from build123d import *

# Parameters (mm, degrees)
SKETCH_1_R          = 20
SKETCH_1_R_2        = 15
EXTRUDE_1_DEPTH     = 4
SKETCH_1_3_R        = 15
EXTRUDE_2_DEPTH     = 15
EXTRUDE_START       = 4
SKETCH_2_R          = 20
EXTRUDE_3_DEPTH     = 4
SKETCH_3_R          = 10
SKETCH_3_R_2        = 4
EXTRUDE_4_DEPTH     = 12
CUT_EXTRUDE_1_DEPTH = 18
CUT_EXTRUDE_START   = -27
SKETCH_3_3_R        = 4
CUT_EXTRUDE_2_DEPTH = 27


with BuildPart() as part:
    # Sketch 1 → Extrude 1 (new body)
    # profile 1 of 2: a face of its own
    with BuildSketch(Plane.XY):
        Circle(SKETCH_1_R)
        Circle(SKETCH_1_R_2, mode=Mode.SUBTRACT)
    # profile 2 of 2: a face of its own
    with BuildSketch(Plane.XY):
        Circle(SKETCH_1_R_2)
    extrude(amount=-EXTRUDE_1_DEPTH)

    # Sketch 1_3 → Extrude 2 (add)
    with BuildSketch(Plane.XY):
        Circle(SKETCH_1_3_R)
    extrude(amount=EXTRUDE_2_DEPTH)

    # Sketch 2 → Extrude 3 (add)
    with BuildSketch(Plane.XY.offset(15).offset(EXTRUDE_START)):
        Circle(SKETCH_2_R)
    extrude(amount=-EXTRUDE_3_DEPTH)

    # Sketch 3 → Extrude 4 (add)
    with BuildSketch(Plane.XY.offset(19)):
        Circle(SKETCH_3_R)
        Circle(SKETCH_3_R_2, mode=Mode.SUBTRACT)
    extrude(amount=EXTRUDE_4_DEPTH)

    # Sketch 4 → Cut-Extrude 1 (cut)
    with BuildSketch(Plane(origin=(0, 0, 0), x_dir=(1, 0, 0), z_dir=(0, 1, 0))):
        with BuildLine():
            ThreePointArc((-1.5, -25), (0, -26.5), (1.5, -25))
            Line((1.5, -25), (-1.5, -25))
        make_face()
        with BuildLine():
            Line((-1.5, -25), (1.5, -25))
            ThreePointArc((1.5, -25), (0, -23.5), (-1.5, -25))
        make_face()
    extrude(amount=CUT_EXTRUDE_1_DEPTH, mode=Mode.SUBTRACT)

    # Sketch 3_3 → Cut-Extrude 2 (cut)
    with BuildSketch(Plane.XY.offset(19).offset(CUT_EXTRUDE_START)):
        Circle(SKETCH_3_3_R)
    extrude(amount=CUT_EXTRUDE_2_DEPTH, mode=Mode.SUBTRACT)


solid = part.part
Verification items for the finished model (mm, model axes). A direction names the side the tool comes from. Coordinates: 2 decimals unless noted, no trailing zeros. Order: outer loops, then holes, each group sorted by start corner. A loop starts at its lowest first (then second) coordinate and runs counter-clockwise, first axis right, second up. Notation, with made-up numbers: M -38.5,43 L -6.5,43 A10 cw -6.5,52 Z; hole C -27,27.5 d4. An arc over 180 degrees is marked long. Return JSON: item names as keys, results as strings.
1) Cross-section at A-A, the plane y = 0. Record the boundary of the cut face in (x, z).
Answer list:
{"outline": "M -20,-4 L -4,-4 L -4,31 L -10,31 L -10,19 L -20,19 L -20,15 L -15,15 L -15,0 L -20,0 Z; M 4,-4 L 20,-4 L 20,0 L 15,0 L 15,15 L 20,15 L 20,19 L 10,19 L 10,31 L 4,31 Z"}
2) Cross-section at D-D, the plane y = -12. Record the boundary of the cut face in (x, z).
Answer list:
{"outline": "M -16,-4 L 16,-4 L 16,0 L 9,0 L 9,15 L 16,15 L 16,19 L -16,19 L -16,15 L -9,15 L -9,0 L -16,0 Z"}
3) Cross-section at B-B, the plane x = -16. Record the boundary of the cut face in (y, z), and give its area (3 significant figures).
Answer list:
{"outline": "M -12,-4 L 12,-4 L 12,0 L -12,0 Z; M -12,15 L 12,15 L 12,19 L -12,19 Z", "area": "192 mm2"}
4) Access from +Z, -Z, +X, -X, +Y, -Y to the whole of each face (thin tool, end or side, straight path). Record for faces 4 (the cylindrical face through (-0.195, 6.811, 23.513)), 5 (the cylindrical face through (-2.17, -9.76, 24.92)), 6 (the cylindrical face through (-14.985, 0.66, 7.395)).
Answer list:
{"face 4": "+Y", "face 5": "+Z", "face 6": "none"}
5) Cross-section at C-C, the plane x = 0. Record the boundary of the cut face in (y, z), and give its area (3 significant figures).
Answer list:
{"outline": "M -20,-4 L -4,-4 L -4,31 L -10,31 L -10,19 L -20,19 L -20,15 L -15,15 L -15,0 L -20,0 Z; M 4,-4 L 20,-4 L 20,0 L 15,0 L 15,15 L 20,15 L 20,19 L 10,19 L 10,23.5 L 4,23.5 Z; M 4,26.5 L 10,26.5 L 10,31 L 4,31 Z", "area": "712 mm2"}
6) Release check for a two-part mould opening along Y. For faces 1 (the cylindrical face through (-0.867, -3.905, 13.255)), 2 (the flat face through (-5, 9, 19)), 3 (the cylindrical face through (-4.336, -19.524, 17.028)) record: +Y half, -Y half, draft (parallel to the pull), parting line (faces both ways), or undercut.
Answer list:
{"face 1": "undercut", "face 2": "draft", "face 3": "parting line"}
7) Gauge pin test, flat ends, axial feed: pin 1 (3 mm diameter, centred on x = 2.5, z = 7.5, fed in from -Y); pin 2 (6 mm diameter, centred on y = -8.5, z = 19.5, fed in from -X); pin 3 (4 mm diameter, centred on x = 14.5, z = 18, fed in from -Y). Record the tip position at first contact, or that the pin passes through.
Answer list:
{"pin 1": "y = -14.97", "pin 2": "x = -19.22", "pin 3": "y = -15.61"}
8) Thickness scan on L1, parallel to Y at x = 0, z = 22.5; L2, parallel to Z at x = -16, y = 6.5; L3, parallel to Z at x = 0, y = 7.25. Record the ranges inside material, lowest first. Write a range as [from, to].
Answer list:
{"L1": "[-10, -4], [4, 10]", "L2": "[-4, 0], [15, 19]", "L3": "[-4, 23.5], [26.5, 31]"}
